```python
from build123d import *

# Parameters (mm, degrees)
SKETCH1_W                      = 110
SKETCH1_H                      = 90
BOSS_EXTRUDE1_DEPTH            = 2.5
M3_CLEARANCE_HOLE1_D           = 3.4
M3_CLEARANCE_HOLE1_DEPTH       = 5
SKETCH5_W                      = 110
SKETCH5_H                      = 6.35
BOSS_EXTRUDE2_DEPTH            = 25
BOSS_EXTRUDE2_DEPTH_BACK       = 2.5
CBORE_FOR_M3_SHCS1_D           = 3.4
CBORE_FOR_M3_SHCS1_DEPTH       = 6.35
CBORE_FOR_M3_SHCS1_CBORE_D     = 6.5
CBORE_FOR_M3_SHCS1_CBORE_DEPTH = 3
CUT_EXTRUDE1_DEPTH             = 6
SKETCH10_W                     = 74.2
SKETCH10_H                     = 70.2
SKETCH10_R                     = 5
SKETCH10_W_2                   = 10
SKETCH10_H_2                   = 15
BOSS_EXTRUDE4_DEPTH            = 5
SKETCH11_W                     = 5
SKETCH11_H                     = 57.74767184
CUT_EXTRUDE2_DEPTH             = 6
FILLET1_R                      = 5


with BuildPart() as part:
    # Sketch1 → Boss-Extrude1 (new body, symmetric)
    with BuildSketch(Plane(origin=(0, 0, 0), x_dir=(1, 0, 0), z_dir=(0, 1, 0))):
        with Locations((55, -45)):
            Rectangle(SKETCH1_W, SKETCH1_H)
    extrude(amount=BOSS_EXTRUDE1_DEPTH, both=True)

    # M3 Clearance Hole1
    with Locations(Plane(origin=(0, 2.5, 0), x_dir=(1, 0, 0), z_dir=(0, 1, 0))):
        with Locations((13.4, -77.55755), (96.6, -12.44245), (96.6, -77.55755), (13.4, -12.44245)):
            Hole(M3_CLEARANCE_HOLE1_D / 2, depth=M3_CLEARANCE_HOLE1_DEPTH)

    # Sketch5 → Boss-Extrude2 (add, two sides)
    with BuildSketch(Plane(origin=(0, 0, 0), x_dir=(1, 0, 0), z_dir=(0, 1, 0))) as boss_extrude2_sk:
        with Locations((55, -93.175)):
            Rectangle(SKETCH5_W, SKETCH5_H)
    extrude(amount=BOSS_EXTRUDE2_DEPTH)
    extrude(boss_extrude2_sk.sketch, amount=-BOSS_EXTRUDE2_DEPTH_BACK)

    # CBORE for M3 SHCS1
    with Locations(Plane(origin=(0, 0, 90), x_dir=(-1, 0, 0), z_dir=(0, 0, -1))):
        with Locations((-80, 13.75), (-30, 13.75)):
            CounterBoreHole(CBORE_FOR_M3_SHCS1_D / 2, CBORE_FOR_M3_SHCS1_CBORE_D / 2, CBORE_FOR_M3_SHCS1_CBORE_DEPTH, depth=CBORE_FOR_M3_SHCS1_DEPTH)

    # Sketch8 → Cut-Extrude1 (cut, through all)
    with BuildSketch(Plane(origin=(0, 2.5, 0), x_dir=(1, 0, 0), z_dir=(0, 1, 0))):
        Polygon((17.9, -9.9), (92.1, -9.9), (92.1, -16.12616408), (100.1, -16.12616408), (100.1, -73.87383592), (92.1, -73.87383592), (92.1, -80.1), (17.9, -80.1), (17.9, -73.87383592), (9.9, -73.87383592), (9.9, -16.12616408), (17.9, -16.12616408), align=None)
    extrude(amount=-CUT_EXTRUDE1_DEPTH, mode=Mode.SUBTRACT)

    # Sketch10 → Boss-Extrude4 (add, through all)
    with BuildSketch(Plane(origin=(0, 2.5, 0), x_dir=(1, 0, 0), z_dir=(0, 1, 0))):
        with Locations((55, -45)):
            Rectangle(SKETCH10_W, SKETCH10_H)
        with Locations((39.76, -57.70755)):
            Circle(SKETCH10_R, mode=Mode.SUBTRACT)
        with Locations((67.7, -57.70755)):
            Circle(SKETCH10_R, mode=Mode.SUBTRACT)
        with Locations((77.1, -25.4)):
            Rectangle(SKETCH10_W_2, SKETCH10_H_2, mode=Mode.SUBTRACT)
    extrude(amount=-BOSS_EXTRUDE4_DEPTH)

    # Sketch11 → Cut-Extrude2 (cut, through all)
    with BuildSketch(Plane(origin=(0, 2.5, 0), x_dir=(1, 0, 0), z_dir=(0, 1, 0))):
        with Locations((20.4, -45)):
            Rectangle(SKETCH11_W, SKETCH11_H)
        with Locations((89.6, -45)):
            Rectangle(SKETCH11_W, SKETCH11_H)
    extrude(amount=-CUT_EXTRUDE2_DEPTH, mode=Mode.SUBTRACT)

    # Fillet1
    fillet1_edges = [part.edges().sort_by_distance(p)[0] for p in [
        (0, 0, 0),
        (110, 0, 0),
        (55, 2.5, 90),
    ]]
    fillet(fillet1_edges, radius=FILLET1_R)


solid = part.part
```
Design review of the part built by this model. Coordinates are the model's own, in mm. A direction names the side the tool comes from. Give positions to 0.01 mm unless a question says otherwise; leave off trailing zeros. Loops run counter-clockwise (first coordinate to the right, second up) from the corner with the lowest first, then second, coordinate; pieces in that order, holes last. Notation, with made-up numbers: M 36.5,-9.5 L 89.5,-9.5 A23 ccw 89.5,14.5 Z; hole C -1,-8.75 d4. An arc over 180 degrees is marked long. Return JSON: item names as keys, results as strings. Group by question number.
Item 1: We need section A-A (z = 51.5). Give the boundary of the cut face in (x, y), and give its area (3 significant figures).
Item 2: We need section C-C (x = 30). Give the boundary of the cut face in (y, z), and give its area (3 significant figures).
Item 3: For probe 1 along Z at (x, y) = (96.6, 0.05); probe 2 along X at (y, z) = (0.75, 31); probe 3 along Y at (x, z) = (80, 94.15), list the stretches that pass through material, from the lowest coordinate up.
Item 4: We need section B-B (x = 13.4). Give the boundary of the cut face in (y, z), and give its area (3 significant figures).
Item 5: We need section D-D (x = 54). Give the boundary of the cut face in (y, z), and give its area (3 significant figures).
Item 6: Mouldability with a two-part tool opening along Y and no side actions: class faces 1 (the cylindrical face through (42.07, 0.04, 62.14)), 2 (the cylindrical face through (55.77, 3.93, 88.5)), 3 (the flat face through (79, 12, 93)) as released by +Y, released by -Y, zero draft, split by the parting line, or undercut.
Item 7: Insertion check: pin 1 Ø1 at (x, y) = (37, 19.5) entering from -Z; pin 2 Ø4 at (x, z) = (82.5, 34) entering from +Y; pin 3 Ø3 at (x, y) = (30.5, 14) entering from -Z. Each pin has a flat end and moves straight along its axis. Give the tip position at first contact, or say it passes through.
Item 8: Tool access review of faces 4 (the flat face through (94, 0, 73.874)), 5 (the flat face through (54, 16, 90)), 6 (the flat face through (29, 12, 93)): name each direction out of +Z, -Z, +X, -X, +Y, -Y from which nothing blocks a thin tool from reaching the whole face with its end or side.
Output:
{
 "1": {"outline": "M 0,-2.5 L 9.9,-2.5 L 9.9,2.5 L 0,2.5 Z; M 22.9,-2.5 L 87.1,-2.5 L 87.1,2.5 L 22.9,2.5 Z; M 100.1,-2.5 L 110,-2.5 L 110,2.5 L 100.1,2.5 Z", "area": "420 mm^2"},
 "2": {"outline": "M -2.5,0 L 2.5,0 L 2.5,85 A5 cw 7.5,90 L 10.5,90 L 10.5,93 L 12.05,93 L 12.05,96.35 L -2.5,96.35 Z; M 15.45,93 L 17,93 L 17,90 L 25,90 L 25,96.35 L 15.45,96.35 Z", "area": "599 mm^2"},
 "3": {"probe 1": "z = 0 to 10.74, 14.14 to 16.13, 73.87 to 75.86, 79.26 to 96.35", "probe 2": "x = 0 to 9.9, 22.9 to 72.1, 82.1 to 87.1, 100.1 to 110", "probe 3": "y = -2.5 to 12.05, 15.45 to 25"},
 "4": {"outline": "M -2.5,0 L 2.5,0 L 2.5,10.74 L -2.5,10.74 Z; M -2.5,14.14 L 2.5,14.14 L 2.5,16.13 L -2.5,16.13 Z; M -2.5,73.87 L 2.5,73.87 L 2.5,75.86 L -2.5,75.86 Z; M -2.5,79.26 L 2.5,79.26 L 2.5,85 A5 cw 7.5,90 L 25,90 L 25,96.35 L -2.5,96.35 Z", "area": "307 mm^2"},
 "5": {"outline": "M -2.5,0 L 2.5,0 L 2.5,85 A5 cw 7.5,90 L 25,90 L 25,96.35 L -2.5,96.35 Z", "area": "630 mm^2"},
 "6": {"face 1": "zero draft", "face 2": "released by +Y", "face 3": "undercut"},
 "7": {"pin 1": "stops at z = 90", "pin 2": "stops at y = 2.5", "pin 3": "stops at z = 93"},
 "8": {"face 4": "+Y, -Y", "face 5": "-Z, +X, -X, +Y", "face 6": "-Z"}
}
